Geometry: final body of the model. Coordinates: model frame, mm. A direction names the side the tool comes from. Round coordinates to 2 decimals unless told otherwise and drop trailing zeros. Loops run counter-clockwise (first coordinate to the right, second up) from the corner with the lowest first, then second, coordinate; pieces in that order, holes last. Notation, with made-up numbers: (-36, 79) -> (3, 79) arc R24 ccw to (3, 118) -> close; hole circle Ø2 at (12, 5.25). An arc over 180 degrees is marked (long way). Answer in a Markdown table with one row per item.
```python
from build123d import *

# Parameters (mm, degrees)
SKETCH1_R           = 47.5
BOSS_EXTRUDE1_DEPTH = 20
SKETCH2_R           = 19.9
BOSS_EXTRUDE2_DEPTH = 65
SKETCH3_R           = 30
BOSS_EXTRUDE3_DEPTH = 30
SKETCH4_R           = 19.9
BOSS_EXTRUDE4_DEPTH = 140
SKETCH5_R           = 7.5
BOSS_EXTRUDE5_DEPTH = 10
SKETCH6_R           = 7
CUT_EXTRUDE1_DEPTH  = 10
SKETCH7_R           = 5
CUT_EXTRUDE2_DEPTH  = 23
SKETCH8_R           = 20
CUT_EXTRUDE3_DEPTH  = 15


with BuildPart() as part:
    # Sketch1 → Boss-Extrude1 (new body)
    with BuildSketch(Plane(origin=(0, 0, 0), x_dir=(1, 0, 0), z_dir=(0, 1, 0))):
        with Locations(Location((0, 0, 0), (0, 0, 270))):
            Circle(SKETCH1_R)
    extrude(amount=BOSS_EXTRUDE1_DEPTH)

    # Sketch2 → Boss-Extrude2 (add)
    with BuildSketch(Plane(origin=(0, 20, 0), x_dir=(1, 0, 0), z_dir=(0, 1, 0))):
        with Locations(Location((0, 0, 0), (0, 0, 270))):
            Circle(SKETCH2_R)
    extrude(amount=BOSS_EXTRUDE2_DEPTH)

    # Sketch3 → Boss-Extrude3 (add)
    with BuildSketch(Plane(origin=(0, 85, 0), x_dir=(1, 0, 0), z_dir=(0, 1, 0))):
        with Locations(Location((0, 0, 0), (0, 0, 270))):
            Circle(SKETCH3_R)
    extrude(amount=BOSS_EXTRUDE3_DEPTH)

    # Sketch4 → Boss-Extrude4 (add)
    with BuildSketch(Plane(origin=(0, 115, 0), x_dir=(1, 0, 0), z_dir=(0, 1, 0))):
        with Locations(Location((0, 0, 0), (0, 0, 270))):
            Circle(SKETCH4_R)
    extrude(amount=BOSS_EXTRUDE4_DEPTH)

    # Sketch5 → Boss-Extrude5 (add)
    with BuildSketch(Plane(origin=(30, 0, 0), x_dir=(0, 0, -1), z_dir=(1, 0, 0))):
        with BuildLine():
            Line((0, 115), (55, 115))
            Line((55, 115), (60, 115))
            ThreePointArc((60, 115), (71.563565439, 106.206860513), (66.180456899, 92.713992392))
            Line((66.180456899, 92.713992392), (53.342217635, 85))
            Line((53.342217635, 85), (0, 85))
            Line((0, 85), (0, 115))
        make_face()
        with Locations((55, 103)):
            Circle(SKETCH5_R, mode=Mode.SUBTRACT)
    boss_extrude5 = extrude(amount=-BOSS_EXTRUDE5_DEPTH)

    # Mirror1: Boss-Extrude5 across plane
    add(boss_extrude5.mirror(Plane(origin=(0, 0, 0), x_dir=(0, 0, 1), z_dir=(1, 0, 0))))

    # Sketch6 → Cut-Extrude1 (cut)
    with BuildSketch(Plane(origin=(0, 20, 0), x_dir=(1, 0, 0), z_dir=(0, 1, 0))):
        with Locations(Location((0, 38, 0), (0, 0, 270))):
            Circle(SKETCH6_R)
        with Locations(Location((38, 0, 0), (0, 0, 270))):
            Circle(SKETCH6_R)
        with Locations(Location((0, -38, 0), (0, 0, 270))):
            Circle(SKETCH6_R)
        with Locations(Location((-38, 0, 0), (0, 0, 270))):
            Circle(SKETCH6_R)
    extrude(amount=-CUT_EXTRUDE1_DEPTH, mode=Mode.SUBTRACT)

    # Sketch7 → Cut-Extrude2 (cut)
    with BuildSketch(Plane.XZ):
        with Locations(Location((0, 38, 0), (0, 0, 270))):
            Circle(SKETCH7_R)
        with Locations(Location((38, 0, 0), (0, 0, 270))):
            Circle(SKETCH7_R)
        with Locations(Location((0, -38, 0), (0, 0, 270))):
            Circle(SKETCH7_R)
        with Locations(Location((-38, 0, 0), (0, 0, 270))):
            Circle(SKETCH7_R)
    extrude(amount=-CUT_EXTRUDE2_DEPTH, mode=Mode.SUBTRACT)

    # Sketch8 → Cut-Extrude3 (cut)
    with BuildSketch(Plane.XZ):
        with Locations(Location((0, 0, 0), (0, 0, 270))):
            Circle(SKETCH8_R)
    extrude(amount=-CUT_EXTRUDE3_DEPTH, mode=Mode.SUBTRACT)


solid = part.part
```
Item 1: Draft query along Y for faces 1 (the face through (25, 89, -60)), 2 (the face through (-2.681, 15.07, -31.534)), 3 (the face through (-19.427, 52.045, -4.314)). Return one class per face: pulls with the +Y half, pulls with the -Y half, needs draft (parallel to the pull), parting line crosses it, or undercut.
Answer:
| item | result |
|---|---|
| face 1 | pulls with the -Y half |
| face 2 | needs draft |
| face 3 | undercut |
Item 2: Pin query (flat end, axial travel): pin 1 Ø19.5 at (y, z) = (103, -55) entering from -X; pin 2 Ø18 at (x, z) = (-38, 0) entering from +Y; pin 3 Ø1.5 at (x, z) = (2, -17.5) entering from -Y; pin 4 Ø8 at (x, z) = (0, -38) entering from -Y. Return the tip coordinate at first contact, or that it passes through.
Answer:
| item | result |
|---|---|
| pin 1 | stops at x = -30 |
| pin 2 | stops at y = 115 |
| pin 3 | stops at y = 15 |
| pin 4 | passes through |
Item 3: Cut plane A-A (x = -38). Output: boundary loops of the cut face in (y, z).
Answer:
| item | result |
|---|---|
| outline | (0, -28.5) -> (20, -28.5) -> (20, -7) -> (10, -7) -> (10, -5) -> (0, -5) -> close; (0, 5) -> (10, 5) -> (10, 7) -> (20, 7) -> (20, 28.5) -> (0, 28.5) -> close |
Item 4: Reachability of faces 4 (the face through (0, 85, -22)), 5 (the face through (-19.524, 7.395, 4.336)), 6 (the face through (30, 100, -29)), 7 (the face through (-30, 100, -29)) from +Z, -Z, +X, -X, +Y, -Y: full face, straight path, thin tool, end or side. Return the list, or none.
Answer:
| item | result |
|---|---|
| face 4 | none |
| face 5 | -Y |
| face 6 | +Z, -Z, +X, +Y |
| face 7 | +Z, -Z, -X, +Y |
Item 5: Cut plane C-C (x = 22.5). Output: boundary loops of the cut face in (y, z).
Answer:
| item | result |
|---|---|
| outline | (0, -41.83) -> (20, -41.83) -> (20, 41.83) -> (0, 41.83) -> close; (85, -53.34) -> (92.71, -66.18) arc R12 ccw to (115, -60) -> (115, 19.84) -> (85, 19.84) -> close; hole circle Ø15 at (103, -55) |
Item 6: Line query: probe 1 along X at (y, z) = (2.25, 0); probe 2 along X at (y, z) = (17.25, 0); probe 3 along Y at (x, z) = (4, 23.5). Output: solid intervals per line, ascending. Write a range as [from, to].
Answer:
| item | result |
|---|---|
| probe 1 | x = [-47.5, -43], [-33, -20], [20, 33], [43, 47.5] |
| probe 2 | x = [-47.5, -45], [-31, 31], [45, 47.5] |
| probe 3 | y = [0, 20], [85, 115] |
Item 7: Cut plane B-B (z = -38). Output: boundary loops of the cut face in (x, y), then the cut area to 3 significant figures.
Answer:
| item | result |
|---|---|
| outline | (-30, 85) -> (-20, 85) -> (-20, 115) -> (-30, 115) -> close; (-28.5, 0) -> (-5, 0) -> (-5, 10) -> (-7, 10) -> (-7, 20) -> (-28.5, 20) -> close; (5, 0) -> (28.5, 0) -> (28.5, 20) -> (7, 20) -> (7, 10) -> (5, 10) -> close; (20, 85) -> (30, 85) -> (30, 115) -> (20, 115) -> close |
| area | 1,500 mm² |
Item 8: Cut plane D-D (z = 22.5). Output: boundary loops of the cut face in (x, y), then the cut area to 3 significant figures.
Answer:
| item | result |
|---|---|
| outline | (-41.83, 0) -> (41.83, 0) -> (41.83, 20) -> (-41.83, 20) -> close; (-19.84, 85) -> (19.84, 85) -> (19.84, 115) -> (-19.84, 115) -> close |
| area | 2,860 mm² |
